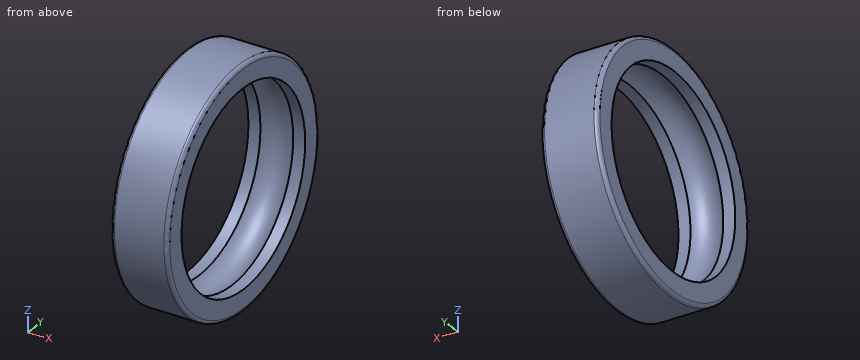
from build123d import *

# Parameters (mm, degrees)
FILLET_1_R = 0.46


with BuildPart() as part:
    # 草图1 → 旋转1 (revolve)
    with BuildSketch(Plane.XY, mode=Mode.PRIVATE) as revolve_1_sk:
        with BuildLine():
            Line((2.061649825, 12.23), (3.575, 12.23))
            Line((3.575, 12.23), (3.575, 15))
            Line((3.575, 15), (-3.575, 15))
            Line((-3.575, 15), (-3.575, 12.23))
            Line((-3.575, 12.23), (-2.061649825, 12.23))
            ThreePointArc((-2.061649825, 12.23), (0, 13.15), (2.061649825, 12.23))
        make_face()
    revolve(revolve_1_sk.sketch.rotate(Axis((0, 0, 0), (1, 0, 0)), 90), axis=Axis((0, 0, 0), (1, 0, 0)))

    # 圆角1
    fillet_1_edges = [part.edges().sort_by_distance(p)[0] for p in [
        (3.575, 0, -15),
        (-3.575, 0, -15),
    ]]
    fillet(fillet_1_edges, radius=FILLET_1_R)


solid = part.part
CAD build for the part. Positions are in the model's coordinates, mm. Round coordinates to 2 decimals unless told otherwise and drop trailing zeros. Loops run counter-clockwise (first coordinate to the right, second up) from the corner with the lowest first, then second, coordinate; pieces in that order, holes last. Notation, with made-up numbers: (78, 25.5) - (127, 25.5) arc R20 ccw to (127, 46.5) - close; hole circle Ø4 at (-2.75, -13.75). An arc over 180 degrees is marked (long way). Put each result on its own line as item: value.
1. Slice it at A-A on y = 0. List the corners of the cut face in (x, z) (3 decimals), and give its area (3 significant figures).
Geometry check:
outline: (-3.575, -14.54) arc R0.46 ccw to (-3.115, -15) - (3.115, -15) arc R0.46 ccw to (3.575, -14.54) - (3.575, -12.23) - (2.062, -12.23) arc R2.77 cw to (-2.062, -12.23) - (-3.575, -12.23) - close; (-3.575, 12.23) - (-2.062, 12.23) arc R2.77 cw to (2.062, 12.23) - (3.575, 12.23) - (3.575, 14.54) arc R0.46 ccw to (3.115, 15) - (-3.115, 15) arc R0.46 ccw to (-3.575, 14.54) - close
area: 34.2 mm²
2. Slice it at D-D on x = 2.75. List the corners of the cut face in (y, z).
Geometry check:
outline: circle Ø30 at (0, 0); hole circle Ø24.46 at (0, 0)
3. Slice it at C-C on x = 0. List the corners of the cut face in (y, z).
Geometry check:
outline: circle Ø30 at (0, 0); hole circle Ø26.3 at (0, 0)
4. Wall check: line 1 (Y direction, x = 3, z = 0); line 2 (Z direction, x = 0.75, y = 7); line 3 (X direction, y = -11.5, z = 5.75) (3 decimals). Give the ranges that are in metal, low to high.
Geometry check:
line 1: -15 to -12.23, 12.23 to 15
line 2: -13.27 to -11.01, 11.01 to 13.27
line 3: -3.575 to -1.239, 1.239 to 3.575
5. Pin check, flat tips, straight feed: P1, Ø4, axis at x = -0.5, y = -2.5, coming from the -Z side; P2, Ø14.5, axis at y = 0, z = 0, coming from the +X side; P3, Ø4, axis at x = -0.5, z = -10, coming from the -Y side; P4, Ø4, axis at x = 0.5, y = -3, coming from the +Z side. Stop position of each tip, or through.
Geometry check:
P1: z = -14.99
P2: through
P3: y = -12.69
P4: z = 14.97
